```python
from build123d import *

# Parameters (mm, degrees)
SKETCH1_R           = 2.5
BOSS_EXTRUDE1_DEPTH = 140
SCALE_2_SCALE       = 3
SCALE_3_SCALE       = 6
SCALE_5_SCALE       = 2
SCALE_6_SCALE       = 0.25
SCALE_7_SCALE       = 0.125
SCALE_8_SCALE       = 0.25
SCALE_9_SCALE       = 4
SCALE_10_SCALE      = 4
OTHER_START         = -17.55
OTHER_1_OUTLINE_R   = 5
OTHER_1_DEPTH       = 10
SKETCH_11_W         = 630
SKETCH_11_H         = 76.5
EXTRUDE_1_DEPTH     = 669


# Read off the part's stored shape, not the designer's step: 孔1
with BuildPart() as part:
    # Sketch1 → Boss-Extrude1 (new body)
    with BuildSketch(Plane.XY):
        with BuildLine():
            Line((2.839339828, 3.9), (5.5, 6.560660172))
            Line((5.5, 6.560660172), (5.5, 8.2))
            Line((5.5, 8.2), (3.1, 8.2))
            Line((3.1, 8.2), (3.1, 9.5))
            Line((3.1, 9.5), (3.6, 9.5))
            Line((3.6, 9.5), (3.6, 10))
            Line((3.6, 10), (8.5, 10))
            ThreePointArc((8.5, 10), (9.560660172, 9.560660172), (10, 8.5))
            Line((10, 8.5), (10, 3.6))
            Line((10, 3.6), (9.5, 3.6))
            Line((9.5, 3.6), (9.5, 3.1))
            Line((9.5, 3.1), (8.2, 3.1))
            Line((8.2, 3.1), (8.2, 5.5))
            Line((8.2, 5.5), (6.560660172, 5.5))
            Line((6.560660172, 5.5), (3.9, 2.839339828))
            Line((3.9, 2.839339828), (3.9, -2.839339828))
            Line((3.9, -2.839339828), (6.560660172, -5.5))
            Line((6.560660172, -5.5), (8.2, -5.5))
            Line((8.2, -5.5), (8.2, -3.1))
            Line((8.2, -3.1), (9.5, -3.1))
            Line((9.5, -3.1), (9.5, -3.6))
            Line((9.5, -3.6), (10, -3.6))
            Line((10, -3.6), (10, -8.5))
            ThreePointArc((10, -8.5), (9.560660172, -9.560660172), (8.5, -10))
            Line((8.5, -10), (3.6, -10))
            Line((3.6, -10), (3.6, -9.5))
            Line((3.6, -9.5), (3.1, -9.5))
            Line((3.1, -9.5), (3.1, -8.2))
            Line((3.1, -8.2), (5.5, -8.2))
            Line((5.5, -8.2), (5.5, -6.560660172))
            Line((5.5, -6.560660172), (2.839339828, -3.9))
            Line((2.839339828, -3.9), (-2.839339828, -3.9))
            Line((-2.839339828, -3.9), (-5.5, -6.560660172))
            Line((-5.5, -6.560660172), (-5.5, -8.2))
            Line((-5.5, -8.2), (-3.1, -8.2))
            Line((-3.1, -8.2), (-3.1, -9.5))
            Line((-3.1, -9.5), (-3.6, -9.5))
            Line((-3.6, -9.5), (-3.6, -10))
            Line((-3.6, -10), (-8.5, -10))
            ThreePointArc((-8.5, -10), (-9.560660172, -9.560660172), (-10, -8.5))
            Line((-10, -8.5), (-10, -3.6))
            Line((-10, -3.6), (-9.5, -3.6))
            Line((-9.5, -3.6), (-9.5, -3.1))
            Line((-9.5, -3.1), (-8.2, -3.1))
            Line((-8.2, -3.1), (-8.2, -5.5))
            Line((-8.2, -5.5), (-6.560660172, -5.5))
            Line((-6.560660172, -5.5), (-3.9, -2.839339828))
            Line((-3.9, -2.839339828), (-3.9, 2.839339828))
            Line((-3.9, 2.839339828), (-6.560660172, 5.5))
            Line((-6.560660172, 5.5), (-8.2, 5.5))
            Line((-8.2, 5.5), (-8.2, 3.1))
            Line((-8.2, 3.1), (-9.5, 3.1))
            Line((-9.5, 3.1), (-9.5, 3.6))
            Line((-9.5, 3.6), (-10, 3.6))
            Line((-10, 3.6), (-10, 8.5))
            ThreePointArc((-10, 8.5), (-9.560660172, 9.560660172), (-8.5, 10))
            Line((-8.5, 10), (-3.6, 10))
            Line((-3.6, 10), (-3.6, 9.5))
            Line((-3.6, 9.5), (-3.1, 9.5))
            Line((-3.1, 9.5), (-3.1, 8.2))
            Line((-3.1, 8.2), (-5.5, 8.2))
            Line((-5.5, 8.2), (-5.5, 6.560660172))
            Line((-5.5, 6.560660172), (-2.839339828, 3.9))
            Line((-2.839339828, 3.9), (2.839339828, 3.9))
        make_face()
        with Locations((0, 0.235847297)):
            Circle(SKETCH1_R, mode=Mode.SUBTRACT)
    extrude(amount=BOSS_EXTRUDE1_DEPTH)


with BuildPart() as part_1:
    # 缩放比例2: scaled about (0, -0.027095247, 70)
    add(part.part.scale(SCALE_2_SCALE).moved(Location((0, 0.054190494, -140))))


with BuildPart() as part_2:
    # 缩放比例3: scaled about (0, -0.027095247, 70)
    add(part_1.part.scale(SCALE_3_SCALE).moved(Location((0, 0.135476235, -350))))


with BuildPart() as part_3:
    # 缩放比例5: scaled about (0, -0.027095249, 70)
    add(part_2.part.scale(SCALE_5_SCALE).moved(Location((0, 0.027095249, -70))))


with BuildPart() as part_4:
    # 缩放比例6: scaled about (0, -0.027095249, 70)
    add(part_3.part.scale(SCALE_6_SCALE).moved(Location((0, -0.020321437, 52.5))))


with BuildPart() as part_5:
    # 缩放比例7: scaled about (0, -0.027095249, 70)
    add(part_4.part.scale(SCALE_7_SCALE).moved(Location((0, -0.023708343, 61.25))))


with BuildPart() as part_6:
    # 缩放比例8: scaled about (0, -0.027095249, 70)
    add(part_5.part.scale(SCALE_8_SCALE).moved(Location((0, -0.020321437, 52.5))))


with BuildPart() as part_7:
    # 缩放比例9: scaled about (0, -0.027095249, 70)
    add(part_6.part.scale(SCALE_9_SCALE).moved(Location((0, 0.081285747, -210))))


with BuildPart() as part_8:
    # 缩放比例10: scaled about (0, -0.027095249, 70)
    add(part_7.part.scale(SCALE_10_SCALE).moved(Location((0, 0.081285747, -210))))

    # 孔1 outline → 孔1 (cut)
    with BuildSketch(Plane.YZ.offset(OTHER_START)):
        with Locations((7.344833538, 1.297306883)):
            Circle(OTHER_1_OUTLINE_R)
    extrude(amount=OTHER_1_DEPTH, mode=Mode.SUBTRACT)

    # 草图11 → 凸台-拉伸1 (add)
    with BuildSketch(Plane(origin=(45, 0, 0), x_dir=(0, 0, -1), z_dir=(1, 0, 0))):
        with Locations((-70, 0.094833365)):
            Rectangle(SKETCH_11_W, SKETCH_11_H)
    extrude(amount=EXTRUDE_1_DEPTH)


solid = part_8.part
```
For this review, take the finished solid that the model builds, in its own axes (mm). A direction names the side the tool comes from. Coordinates: 2 decimals unless noted, no trailing zeros. Order: outer loops, then holes, each group sorted by start corner. A loop starts at its lowest first (then second) coordinate and runs counter-clockwise, first axis right, second up. Notation, with made-up numbers: (66, 49) -> (92, 49) arc R29 cw to (92, 79) -> close; hole circle Ø10 at (83, -2.5). An arc over 180 degrees is marked (long way). Answer as CSV lines item,"result".
Q1. Clearance check with flat-ended pins moving along their axes: pin 1 Ø1.1 at (x, z) = (15.5, 35.5) entering from -Y; pin 2 Ø4 at (x, z) = (412.5, 264) entering from -Y; pin 3 Ø1.8 at (x, z) = (40, 36) entering from +Y. State where each tip first meets the part, or that it passes through.
Model answer:
pin 1,"stops at y = -42.66"
pin 2,"stops at y = -38.16"
pin 3,"stops at y = 45.04"
Q2. For faces 1 (the face through (375, 38.345, 74)), 2 (the face through (375, -38.155, 74)), 3 (the face through (0, -17.455, 66)), 4 (the face through (-17.55, 0, 66)), 5 (the face through (45, 0, 74)), list the 3-axis set-ups (+Z, -Z, +X, -X, +Y, -Y) from which the entire face can be reached by the end or side of a thin tool; tool diameter is ignored.
Model answer:
face 1,"+Z, -Z, +X, +Y"
face 2,"+Z, -Z, +X, -Y"
face 3,"+Z, -Z, -Y"
face 4,"+Z, -Z, -X"
face 5,"+Z, -Z"
Q3. We need section A-A (x = 551). State the section outline as (y, z) points.
Model answer:
outline,"(-38.16, -245) -> (38.34, -245) -> (38.34, 385) -> (-38.16, 385) -> close"
Q4. Draft analysis for pull direction Y (two halves, no side actions). For faces 6 (the face through (714, 1, 74)), 7 (the face through (17.55, 0, 66)), 8 (the face through (0, 17.645, 66)), state which applies: released by +Y, released by -Y, zero draft, split by the parting line, or undercut.
Model answer:
face 6,"zero draft"
face 7,"undercut"
face 8,"released by +Y"
Q5. We need section B-B (z = 153). Count the separate pieces of the cut face and the enclosed holes in it, plus the area to 3 significant figures.
Model answer:
separate pieces,"1"
enclosed holes,"2"
area,"54,600 mm2"
Q6. Wall thickness on line 1 along X through (y, z) = (-31, -80); line 2 along X through (y, z) = (0, 203); line 3 along Y through (x, z) = (0, 161.5): over which ranges is each line inside the solid? List them lowest first. Write a range as [from, to].
Model answer:
line 1,"x = [-45, -24.75], [24.75, 714]"
line 2,"x = [-17.55, -11.19], [11.19, 17.55], [45, 714]"
line 3,"y = [-17.46, -10.09], [12.41, 17.64]"
